Source: CAD feature listing. Evaluate the final solid. Frame: model axes, mm. A direction names the side the tool comes from. Give positions to 0.01 mm unless a question says otherwise; leave off trailing zeros. Order: outer loops, then holes, each group sorted by start corner. A loop starts at its lowest first (then second) coordinate and runs counter-clockwise, first axis right, second up.
from build123d import *

# Parameters (mm, degrees)
SKETCH_1_W          = 30
SKETCH_1_H          = 38
EXTRUDE_1_DEPTH     = 3
SKETCH_2_W          = 30
SKETCH_2_H          = 3
EXTRUDE_2_DEPTH     = 35
SKETCH_3_R          = 1.5
CUT_EXTRUDE_1_DEPTH = 35
SKETCH_4_R          = 1.5
CUT_EXTRUDE_2_DEPTH = 35


with BuildPart() as part:
    # 草图1 → 凸台-拉伸1 (new body)
    with BuildSketch(Plane.XY):
        Rectangle(SKETCH_1_W, SKETCH_1_H)
    extrude(amount=EXTRUDE_1_DEPTH)

    # 草图2 → 凸台-拉伸2 (add)
    with BuildSketch(Plane.XY.offset(3)):
        with Locations((0, -17.5)):
            Rectangle(SKETCH_2_W, SKETCH_2_H)
    extrude(amount=EXTRUDE_2_DEPTH)

    # 草图3 → 切除-拉伸1 (cut)
    with BuildSketch(Plane.XY.offset(3)):
        with Locations((-10, 4)):
            Circle(SKETCH_3_R)
        with Locations((10, 4)):
            Circle(SKETCH_3_R)
    extrude(amount=-CUT_EXTRUDE_1_DEPTH, mode=Mode.SUBTRACT)

    # 草图4 → 切除-拉伸2 (cut)
    with BuildSketch(Plane(origin=(0, -16, 0), x_dir=(1, 0, 0), z_dir=(0, 1, 0))):
        with Locations(Location((-10, -23, 0), (0, 0, 270))):
            Circle(SKETCH_4_R)
        with Locations(Location((10, -23, 0), (0, 0, 270))):
            Circle(SKETCH_4_R)
    extrude(amount=-CUT_EXTRUDE_2_DEPTH, mode=Mode.SUBTRACT)


solid = part.part
1) Pull-direction query (Y, two-part tool) for faces 3 (the face through (-11.5, 4.07, 1.52)), 4 (the face through (10.07, -17.48, 21.5)), 5 (the face through (0, -16, 20)), 6 (the face through (8.5, 4.07, 1.52)); classes: +Y half, -Y half, draft (parallel to the pull), parting line (faces both ways), or undercut.
Checks:
face 3: undercut
face 4: draft
face 5: +Y half
face 6: undercut
2) Section query B-B on y = 4. Output: boundary loops of the cut face in (x, z).
Checks:
outline: (-15, 0) - (-11.5, 0) - (-11.5, 3) - (-15, 3) - close; (-8.5, 0) - (8.5, 0) - (8.5, 3) - (-8.5, 3) - close; (11.5, 0) - (15, 0) - (15, 3) - (11.5, 3) - close
3) Section query D-D on x = 5. Output: boundary loops of the cut face in (y, z), and give its area (3 significant figures).
Checks:
outline: (-19, 0) - (19, 0) - (19, 3) - (-16, 3) - (-16, 38) - (-19, 38) - close
area: 219 mm2
4) Section query A-A on z = 23. Output: boundary loops of the cut face in (x, y).
Checks:
outline: (-15, -19) - (-11.5, -19) - (-11.5, -16) - (-15, -16) - close; (-8.5, -19) - (8.5, -19) - (8.5, -16) - (-8.5, -16) - close; (11.5, -19) - (15, -19) - (15, -16) - (11.5, -16) - close
5) Section query C-C on x = 10. Output: boundary loops of the cut face in (y, z).
Checks:
outline: (-19, 0) - (2.5, 0) - (2.5, 3) - (-16, 3) - (-16, 21.5) - (-19, 21.5) - close; (-19, 24.5) - (-16, 24.5) - (-16, 38) - (-19, 38) - close; (5.5, 0) - (19, 0) - (19, 3) - (5.5, 3) - close
6) Reachability of faces 1 (the face through (0, 19, 1)), 2 (the face through (0, 2, 3)) from +Z, -Z, +X, -X, +Y, -Y: full face, straight path, thin tool, end or side. Return the list, or none.
Checks:
face 1: +Z, -Z, +X, -X, +Y
face 2: +Z, +X, -X, +Y
7) First-contact query: pin 1 Ø15 at (x, z) = (6, 18.5) entering from +Y; pin 2 Ø8 at (x, y) = (-1.5, -4) entering from +Z. Flat tips, straight axial feed; report the tip coordinate or a pass-through.
Checks:
pin 1: stops at y = -16
pin 2: stops at z = 3
8) Ray query, L1, parallel to Y at x = -10, z = 2; L2, parallel to Y at x = -11, z = 26; L3, parallel to Z at x = -1.5, y = -0.5. Return the intervals inside material, ascending.
Checks:
L1: y = -19 to 2.5, 5.5 to 19
L2: y = -19 to -16
L3: z = 0 to 3
